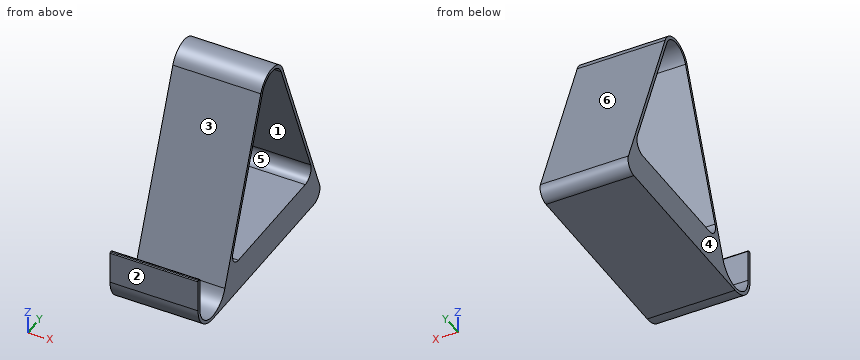
from build123d import *

# Parameters (mm, degrees)
F1_DEPTH = 40


with BuildPart() as f1:
    # F0 (on Right) → F1 (new body)
    with BuildSketch(Plane.YZ):
        with BuildLine():
            Line((-12.5, 14.6), (-12.5, 0))
            ThreePointArc((-12.5, 0), (-8.838835, -8.838835), (0, -12.5))
            Line((0, -12.5), (85.754689, -12.5))
            ThreePointArc((85.754689, -12.5), (89.885373, -10.317348), (90.409718, -5.674979))
            Line((90.409718, -5.674979), (59.310059, 73.650042))
            ThreePointArc((59.310059, 73.650042), (50, 80), (40.689941, 73.650042))
            Line((40.689941, 73.650042), (10.241065, -4.015046))
            ThreePointArc((10.241065, -4.015046), (-2.043072, -10.808601), (-11, 0))
            Line((-11, 0), (-11, 14.6))
            ThreePointArc((-11, 14.6), (-11.117157, 14.882843), (-11.4, 15))
            Line((-11.4, 15), (-12.1, 15))
            ThreePointArc((-12.1, 15), (-12.382843, 14.882843), (-12.5, 14.6))
        make_face()
        with BuildLine():
            ThreePointArc((42.08645, 73.102536), (50, 78.5), (57.91355, 73.102536))
            Line((57.91355, 73.102536), (82.917754, 9.325021))
            ThreePointArc((82.917754, 9.325021), (82.393408, 4.682652), (78.262724, 2.5))
            Line((78.262724, 2.5), (21.737276, 2.5))
            ThreePointArc((21.737276, 2.5), (17.606592, 4.682652), (17.082246, 9.325021))
            Line((17.082246, 9.325021), (42.08645, 73.102536))
        make_face(mode=Mode.SUBTRACT)
    extrude(amount=-F1_DEPTH)


solid = f1.part
The listing builds one solid part. Answer for the finished solid, in the listing's coordinates (mm). Face numbers are marked on the shaded views. A direction names the side the tool comes from. Round coordinates to 2 decimals unless told otherwise and drop trailing zeros. Write each loop counter-clockwise with the first axis right and the second up, starting at its lowest first coordinate (ties: lowest second). Pieces come first, ordered by that corner, then holes. Notation, with made-up numbers: M -13,-24 L 46,-24 A23 cw 46,1 Z; hole C 88.25,33.25 d3. An arc over 180 degrees is marked long. Write each question's results on one line, items separated by ' | '. Start each with the question number.
Item 1: A cutting plane is placed at C-C on z = 69.5. Write down the section's boundary in (x, y).
Item 2: For a pull along Y with two mould halves and no side action, classify the marked faces 4, 5 and 6 as pulls with the +Y half, pulls with the -Y half, needs draft (parallel to the pull), parting line crosses it, or undercut.
Item 3: For the marked faces 1, 2 and 3, determine the directions among +Z, -Z, +X, -X, +Y, -Y from which every point of the face is accessible in a straight line to the end or side of a thin tool.
Item 4: Straight lines are drawn through the part: L1, parallel to Y at x = -32.5, z = 74; L2, parallel to Y at x = -12.5, z = -9; L3, parallel to Y at x = -30, z = 4.5. For each, find the intervals that lie inside material, in ascending order. Write a range as [from, to].
Item 5: Flat-ended cylindrical pins translate along their axes: pin 1 Ø12 at (x, z) = (-17, 68.5) entering from -Y; pin 2 Ø11.5 at (x, z) = (-27, 5) entering from +Y; pin 3 Ø1 at (x, z) = (-35, 37) entering from +Y. Find the tip coordinate at first contact, or state that the pin passes through.
Item 6: A cutting plane is placed at B-B on y = 60.5. Write down the section's boundary in (x, z), and give its area (3 significant figures).
Item 7: A cutting plane is placed at A-A on x = -15. Write down the section's boundary in (y, z), and give its area (3 significant figures).
Check sheet entries:
1) outline: M -40,39.06 L 0,39.06 L 0,40.67 L -40,40.67 Z; M -40,59.33 L 0,59.33 L 0,60.94 L -40,60.94 Z
2) face 4: needs draft | face 5: undercut | face 6: pulls with the +Y half
3) face 1: +X, -X | face 2: +Z, -Z, +X, -X, -Y | face 3: +Z, +X, -X
4) L1: [40.83, 42.5], [57.5, 59.17] | L2: [-8.67, -6.32], [6.32, 90.52] | L3: [-12.5, -11], [13.58, 17.74], [82.26, 86.42]
5) pin 1: y = 36.32 | pin 2: y = 88.48 | pin 3: y = 73.87
6) outline: M -40,-12.5 L 0,-12.5 L 0,2.5 L -40,2.5 Z; M -40,66.51 L 0,66.51 L 0,70.61 L -40,70.61 Z | area: 764 mm²
7) outline: M -12.5,0 A12.5 ccw 0,-12.5 L 85.75,-12.5 A5 ccw 90.41,-5.67 L 59.31,73.65 A10 ccw 40.69,73.65 L 10.24,-4.02 A11 cw -11,0 L -11,14.6 A0.4 ccw -11.4,15 L -12.1,15 A0.4 ccw -12.5,14.6 Z; hole M 17.08,9.33 A5 ccw 21.74,2.5 L 78.26,2.5 A5 ccw 82.92,9.33 L 57.91,73.1 A8.5 ccw 42.09,73.1 Z | area: 1,550 mm²
